Could you check a few things on this model? Use its own coordinates, in mm. A direction names the side the tool comes from. Round coordinates to 2 decimals unless told otherwise and drop trailing zeros. Loops run counter-clockwise (first coordinate to the right, second up) from the corner with the lowest first, then second, coordinate; pieces in that order, holes last. Notation, with made-up numbers: (-9, 64) -> (2, 64) arc R24 cw to (2, 97) -> close; hole circle Ø2 at (-11, -19.75). An arc over 180 degrees is marked (long way). Put each result on its own line as item: value. Start each with the question number.
1. Imagine slicing it at C-C, the plane z = 2. Please give me the cut outline in (x, y).
2. Imagine slicing it at D-D, the plane y = -9.5. Please give me the cut outline in (x, z).
3. I need wall thicknesses on line 1 (Y direction, x = 19.75, z = 6.4); line 2 (X direction, y = -9.5, z = 4.9); line 3 (X direction, y = 9.5, z = 0.7). Which ranges of each line are inside material? Lowest first, please. Write a range as [from, to].
4. Imagine slicing it at B-B, the plane x = 19.75. Please give me the cut outline in (y, z), and give its area (3 significant figures).
5. If we mould it in two halves opening along X, with no side actions, what happens to faces 1 (the flat face through (25, 0, 4)), 2 (the flat face through (20, 0, 8)), 3 (the flat face through (-10, 12, 3)), 4 (the cylindrical face through (17.767, -9.76, 5.535))? For each: pulls with the +X half, pulls with the -X half, needs draft (parallel to the pull), parting line crosses it, or undercut.
6. I'm going to push flat-ended pins straight in: P1, Ø8, axis at x = -9, y = 2, coming from the +Z side; P2, Ø3.5, axis at x = -19, y = 9.5, coming from the -Z side; P3, Ø3, axis at x = -4, z = 3, coming from the +Y side. Where does each tip first touch, or does it pass through?
7. Imagine slicing it at A-A, the plane y = -0.75. Please give me the cut outline in (x, z), and give its area (3 significant figures).
8. Which directions (+Z, -Z, +X, -X, +Y, -Y) give clear straight access to the entire face, cutting with the end or side of a thin tool? Please do faces 5 (the flat face through (0, -11.5, 3)), 6 (the cylindrical face through (-23.22, -9.96, 1.52)), 7 (the flat face through (16.5, 12, 6.9)).
Autodesk Inventor part; units mm, degrees
ref_plane "YZ Plane" through (0, 0, 0) normal (1, 0, 0) x (0, 1, 0)
ref_plane "XZ Plane" through (0, 0, 0) normal (0, 1, 0) x (-1, 0, 0)
ref_plane "XY Plane" through (0, 0, 0) normal (0, 0, 1) x (1, 0, 0)
sketch "Sketch1" plane through (0, 0, 0) normal (0, 0, 1) x (1, 0, 0)
  line L0 (-25, 13.5) -> (25, 13.5)
  line L1 (25, 13.5) -> (25, -13.5)
  line L2 (25, -13.5) -> (-25, -13.5)
  line L3 (-25, -13.5) -> (-25, 13.5)
  point P0 (0, 0)
  point P1 (0, 13.5)
  point P2 (-25, 0)
  dimension "d0" = 27
  dimension "d1" = 50
extrude "Extrusion1" add sketch "Sketch1" along normal blind 8
sketch "Sketch2" plane through (0, 0, 8) normal (0, 0, 1) x (1, 0, 0)
  arc A0 (-10.3042, 3.1624) -> (-9.6648, 2.3936) centre (-9.9845, 2.778) ccw
  line L0 (-1.0786, 10.8363) -> (-10.3042, 3.1624)
  arc A1 (-0.4391, 10.0675) -> (-1.0786, 10.8363) centre (-0.7589, 10.4519) ccw
  line L1 (-9.6648, 2.3936) -> (-0.4391, 10.0675)
  arc A2 (-9.156, -1.3455) -> (-8.5165, -2.1143) centre (-8.8363, -1.7299) ccw
  line L2 (3.1448, 8.8863) -> (-9.156, -1.3455)
  arc A3 (3.7843, 8.1175) -> (3.1448, 8.8863) centre (3.4646, 8.5019) ccw
  line L3 (-8.5165, -2.1143) -> (3.7843, 8.1175)
  arc A4 (-8.0078, -5.8535) -> (-7.3683, -6.6223) centre (-7.688, -6.2379) ccw
  line L4 (7.3683, 6.9363) -> (-8.0078, -5.8535)
  arc A5 (8.0078, 6.1675) -> (7.3683, 6.9363) centre (7.688, 6.5519) ccw
  line L5 (-7.3683, -6.6223) -> (8.0078, 6.1675)
  arc A6 (-3.7843, -7.8035) -> (-3.1448, -8.5723) centre (-3.4646, -8.1879) ccw
  line L6 (8.5165, 2.4283) -> (-3.7843, -7.8035)
  arc A7 (9.156, 1.6595) -> (8.5165, 2.4283) centre (8.8363, 2.0439) ccw
  line L7 (-3.1448, -8.5723) -> (9.156, 1.6595)
  arc A8 (0.4391, -9.7535) -> (1.0786, -10.5223) centre (0.7589, -10.1379) ccw
  line L8 (9.6648, -2.0796) -> (0.4391, -9.7535)
  arc A9 (10.3042, -2.8484) -> (9.6648, -2.0796) centre (9.9845, -2.464) ccw
  line L9 (1.0786, -10.5223) -> (10.3042, -2.8484)
  line L10 (9.5, 13.5) -> (-9.5, 13.5)
  line L11 (-9.5, 13.5) -> (-9.5, -11.5)
  line L12 (-9.5, -11.5) -> (9.5, -11.5)
  line L13 (9.5, -11.5) -> (9.5, 13.5)
  line L14 (-25, -13.5) -> (25, -13.5)
  line L15 (25, 13.5) -> (-25, 13.5)
  point P0 (0, 0)
  point P1 (0, -11.5)
  point P2 (0, -13.5)
  dimension "d4" = 19
  dimension "d5" = 2
extrude "Extrusion2" cut sketch "Sketch2" against normal through all contours L11 L10 L13 L8 A8 L9 L12 L1 A1 L0 | L0 A1 L1 L11 | L13 L9 A8 L8 | L2 A3 L3 A2 | L4 A5 L5 A4 | L6 A7 L7 A6
sketch "Sketch3" plane through (0, 0, 8) normal (0, 0, 1) x (1, 0, 0)
  line L0 (9.5, 13.5) -> (9.5, -11.5)
  line L1 (9.5, -11.5) -> (-9.5, -11.5)
  line L2 (-9.5, -11.5) -> (-9.5, 13.5)
  line L3 (9.5, 13.5) -> (16, 13.5)
  line L4 (25, 13.5) -> (9.5, 13.5)
  line L5 (16, 13.5) -> (16, -16.5)
  line L6 (16, -16.5) -> (-16, -16.5)
  line L7 (-16, -16.5) -> (-16, 13.5)
  line L8 (-9.5, 13.5) -> (-25, 13.5)
  circle A0 centre (0, 0.157) radius 12.5
  point P0 (0, 0)
  dimension "d8" = 6.5
  dimension "d9" = 6.5
  dimension "d10" = 5
extrude "Extrusion3" cut sketch "Sketch3" against normal blind 2.3 contours L3 L5 L6 L7 L8 L2 A0 L1 L0 | A0 L0 | L2 A0 | A0 L1
sketch "Sketch4" plane through (0, 0, 0) normal (0, 0, -1) x (-1, 0, 0)
  line L0 (-25, -13.5) -> (-25, 13.5)
  line L1 (-25, 13.5) -> (-9.5, 13.5)
  line L2 (25, -13.5) -> (-25, -13.5)
  point P0 (0, 0)
  point P1 (-19.75, 9.5)
  point P2 (-19.75, -9.5)
  dimension "d13" = 5.25
  dimension "d14" = 4
  dimension "d15" = 4
hole "Hole1" at (19.75, 9.5, 0) at (19.75, -9.5, 0) direction (0, 0, 1) diameter 4 depth 8 tip angle 118 counterbore diameter 7 counterbore depth 3
mirror "Mirror1" about plane through (0, 0, 0) normal (1, 0, 0) of "Hole1"
chamfer "Chamfer1" distance 1 distance2 3 1 edges at (9.5, 13.5, 2.85) measured on face at (16.8333, 13.5, 1.9)
chamfer "Chamfer2" distance 1 distance2 3 1 edges at (16, 13.5, 6.85) measured on face at (17.1667, 13.5, 1.9)
chamfer "Chamfer3" distance 1 distance2 3 1 edges at (-9.5, 13.5, 2.85) measured on face at (-16.8333, 13.5, 1.9)
chamfer "Chamfer4" distance 1 distance2 3 1 edges at (-16, 13.5, 6.85) measured on face at (-17.1667, 13.5, 1.9)
equation "\"d9\" = d8"
properties part number "0008-10-003"
Entries:
1. outline: (-25, -13.5) -> (25, -13.5) -> (25, 13.5) -> (10.5, 13.5) -> (9.5, 10.5) -> (9.5, -11.5) -> (-9.5, -11.5) -> (-9.5, 10.5) -> (-10.5, 13.5) -> (-25, 13.5) -> close; hole circle Ø7 at (-19.75, -9.5); hole circle Ø7 at (-19.75, 9.5); hole circle Ø7 at (19.75, -9.5); hole circle Ø7 at (19.75, 9.5)
2. outline: (-25, 0) -> (-23.25, 0) -> (-23.25, 3) -> (-21.75, 3) -> (-21.75, 8) -> (-25, 8) -> close; (-17.75, 3) -> (-16.25, 3) -> (-16.25, 0) -> (-9.5, 0) -> (-9.5, 5.7) -> (-16, 5.7) -> (-16, 8) -> (-17.75, 8) -> close; (9.5, 0) -> (16.25, 0) -> (16.25, 3) -> (17.75, 3) -> (17.75, 8) -> (16, 8) -> (16, 5.7) -> (9.5, 5.7) -> close; (21.75, 3) -> (23.25, 3) -> (23.25, 0) -> (25, 0) -> (25, 8) -> (21.75, 8) -> close
3. line 1: [-13.5, -11.5], [-7.5, 7.5], [11.5, 13.5]
3. line 2: [-25, -21.75], [-17.75, -9.5], [9.5, 17.75], [21.75, 25]
3. line 3: [-25, -23.25], [-16.25, -9.5], [9.5, 16.25], [23.25, 25]
4. outline: (-13.5, 0) -> (-13, 0) -> (-13, 3) -> (-11.5, 3) -> (-11.5, 8) -> (-13.5, 8) -> close; (-7.5, 3) -> (-6, 3) -> (-6, 0) -> (6, 0) -> (6, 3) -> (7.5, 3) -> (7.5, 8) -> (-7.5, 8) -> close; (11.5, 3) -> (13, 3) -> (13, 0) -> (13.5, 0) -> (13.5, 8) -> (11.5, 8) -> close
4. area: 134 mm^2
5. face 1: pulls with the +X half
5. face 2: needs draft
5. face 3: undercut
5. face 4: undercut
6. P1: z = 5.7
6. P2: z = 3
6. P3: y = -11.5
7. outline: (-25, 0) -> (-9.5, 0) -> (-9.5, 5.7) -> (-16, 5.7) -> (-16, 8) -> (-25, 8) -> close; (9.5, 0) -> (25, 0) -> (25, 8) -> (16, 8) -> (16, 5.7) -> (9.5, 5.7) -> close
7. area: 218 mm^2
8. face 5: +Z, -Z, +Y
8. face 6: -Z
8. face 7: +Z, +Y
